from build123d import *

# Parameters (mm, degrees)
EXTRUDE_1_DEPTH = 2
SKETCH_2_W      = 3
SKETCH_2_H      = 3
EXTRUDE_2_DEPTH = 10


with BuildPart() as part:
    # 스케치1 → 보스-돌출1 (new body)
    with BuildSketch(Plane(origin=(0, 0, 0), x_dir=(1, 0, 0), z_dir=(0, 1, 0))):
        Polygon((3.23, 0), (1.615, 2.797262054), (-1.615, 2.797262054), (-3.23, 0), (-1.615, -2.797262054), (1.615, -2.797262054), align=None)
    extrude(amount=EXTRUDE_1_DEPTH)

    # 스케치2 → 보스-돌출2 (add)
    with BuildSketch(Plane(origin=(0, 2, 0), x_dir=(1, 0, 0), z_dir=(0, 1, 0))):
        Rectangle(SKETCH_2_W, SKETCH_2_H)
    extrude(amount=EXTRUDE_2_DEPTH)


solid = part.part
Design review of the part built by this model. Coordinates are the model's own, in mm. A direction names the side the tool comes from. Round coordinates to 2 decimals unless told otherwise and drop trailing zeros. Order: outer loops, then holes, each group sorted by start corner. A loop starts at its lowest first (then second) coordinate and runs counter-clockwise, first axis right, second up. Notation, with made-up numbers: M 66,72.5 L 114,72.5 A26 cw 114,87.5 Z; hole C 35.5,87 d8. An arc over 180 degrees is marked long. Answer as CSV lines item,"result". Start each with the question number.
1) Tool access review of faces 1 (the face through (1.5, 7, 0)), 2 (the face through (-1.5, 7, 0)), 3 (the face through (0, 7, -1.5)): name each direction out of +Z, -Z, +X, -X, +Y, -Y from which nothing blocks a thin tool from reaching the whole face with its end or side.
2) Add section C-C (z = -0.2). Give the boundary of the cut face in (x, y).
3) Add section B-B (y = 1). Give the boundary of the cut face in (x, z) (3 decimals), then the cut area to 3 significant figures.
4) Wall thickness on line 1 along Y through (x, z) = (-1.25, 2.3); line 2 along Z through (x, y) = (0.75, 5): over which ranges is each line inside the solid? List them lowest first. Write a range as [from, to].
5) Add section D-D (y = 8). Give the boundary of the cut face in (x, z), then the cut area to 3 significant figures.
6) For pin 1 Ø1.5 at (x, y) = (-0.5, 6) entering from -Z; pin 2 Ø2.5 at (x, y) = (0, 5.5) entering from +Z; pin 3 Ø2.5 at (y, z) = (7, 0.5) entering from +X, all flat-tipped, find the tip position at first contact; note any pin that passes through.
7) Add section A-A (x = -0.75). Give the boundary of the cut face in (y, z), then the cut area to 3 significant figures.
Resolved:
1,face 1,"+Z, -Z, +X, +Y"
1,face 2,"+Z, -Z, -X, +Y"
1,face 3,"-Z, +X, -X, +Y"
2,outline,"M -3.11,0 L 3.11,0 L 3.11,2 L 1.5,2 L 1.5,12 L -1.5,12 L -1.5,2 L -3.11,2 Z"
3,outline,"M -3.23,0 L -1.615,-2.797 L 1.615,-2.797 L 3.23,0 L 1.615,2.797 L -1.615,2.797 Z"
3,area,"27.1 mm^2"
4,line 1,"[0, 2]"
4,line 2,"[-1.5, 1.5]"
5,outline,"M -1.5,-1.5 L 1.5,-1.5 L 1.5,1.5 L -1.5,1.5 Z"
5,area,"9.00 mm^2"
6,pin 1,"z = -1.5"
6,pin 2,"z = 1.5"
6,pin 3,"x = 1.5"
7,outline,"M 0,-2.8 L 2,-2.8 L 2,-1.5 L 12,-1.5 L 12,1.5 L 2,1.5 L 2,2.8 L 0,2.8 Z"
7,area,"41.2 mm^2"
